Autodesk Inventor part; units mm, degrees
ref_plane "YZ Plane" through (0, 0, 0) normal (1, 0, 0) x (0, 1, 0)
ref_plane "XZ Plane" through (0, 0, 0) normal (0, 1, 0) x (-1, 0, 0)
ref_plane "XY Plane" through (0, 0, 0) normal (0, 0, 1) x (1, 0, 0)
sketch "Boceto1" plane through (0, 0, 0) normal (0, 0, 1) x (1, 0, 0)
  line L0 (0.15, 0) -> (0, 0)
  line L1 (0, 0) -> (0, 8.5)
  line L2 (0, 8.5) -> (0.15, 8.5)
  line L3 (0.15, 8.5) -> (0.15, 0)
  line L4 (0.15, 0) -> (5.9, 0)
  line L5 (5.9, 0) -> (5.9, 8.5)
  line L6 (5.9, 8.5) -> (5.75, 8.5)
  line L7 (5.75, 8.5) -> (5.6932, 0)
  line L8 (5.75, 8.5) -> (0.15, 8.5)
  circle A0 centre (0.5, 2.35) radius 0.15
  circle A1 centre (5.4, 2.35) radius 0.15
  circle A2 centre (0.5, 8.15) radius 0.15
  circle A3 centre (5.4, 8.15) radius 0.15
extrude "Extrusión1" add sketch "Boceto1" along normal blind 0.15
sketch "Boceto2" plane through (5.9, 0, 0) normal (1, 0, 0) x (0, 0, -1)
  line L0 (0, 0) -> (0, 8.5)
  line L1 (0, 8.5) -> (-0.8328, 8.5)
  line L2 (-0.8328, 8.5) -> (-0.8328, 0)
  line L3 (-0.8328, 0) -> (0, 0)
  circle A0 centre (-0.3164, 0.3) radius 0.15
  circle A1 centre (-0.3164, 1.2) radius 0.15
  line L4 (0, 8.5) -> (-0.15, 8.5)
  line L5 (-0.15, 8.5) -> (-0.15, 0)
extrude "Extrusión2" add sketch "Boceto2" against normal blind 0.15 contours L3 L2 L1 L5
sketch "Boceto3" plane through (0, 0, 0) normal (-1, 0, 0) x (0, 0, 1)
  line L0 (0, 0) -> (0, 8.5)
  line L1 (0, 8.5) -> (0.8328, 8.5)
  line L2 (0.8328, 8.5) -> (0.8328, 0)
  line L3 (0.8328, 0) -> (0, 0)
  circle A0 centre (0.3164, 0.3) radius 0.15
  circle A1 centre (0.3164, 1.2) radius 0.15
  line L4 (0, 8.5) -> (0.15, 8.5)
  line L5 (0.15, 8.5) -> (0.15, 0)
extrude "Extrusión3" add sketch "Boceto3" against normal blind 0.15 contours L5 L1 L2 L3
properties part number "learnbotAgarreOdroid"
Geometry: final body of the model. Coordinates: model frame, mm. Round coordinates to 2 decimals unless told otherwise and drop trailing zeros. Write each loop counter-clockwise with the first axis right and the second up, starting at its lowest first coordinate (ties: lowest second). Pieces come first, ordered by that corner, then holes. Notation, with made-up numbers: M 13.5,-34 L 49.5,-34 A27 ccw 49.5,-12 Z; hole C -6.5,38.25 d9. An arc over 180 degrees is marked long. Write item = value, one per line.
Item 1: Material intervals for line 1 along X through (y, z) = (2.5, 0.75); line 2 along Y through (x, z) = (5.4, 0.1); line 3 along Z through (x, y) = (0.7, 2.75), sorted ascending. Write a range as [from, to].
Findings:
line_1 = [0, 0.15], [5.75, 5.9]
line_2 = [0, 2.2], [2.5, 8], [8.3, 8.5]
line_3 = [0, 0.15]
Item 2: Section query B-B on x = 0.5. Return loops of the section in (y, z), then the cut area to 4 significant figures.
Findings:
outline = M 0,0 L 2.2,0 L 2.2,0.15 L 0,0.15 Z; M 2.5,0 L 8,0 L 8,0.15 L 2.5,0.15 Z; M 8.3,0 L 8.5,0 L 8.5,0.15 L 8.3,0.15 Z
area = 1.185 mm^2
Item 3: Section query C-C on y = 7. Return loops of the section in (x, z).
Findings:
outline = M 0,0 L 5.9,0 L 5.9,0.83 L 5.75,0.83 L 5.75,0.15 L 0.15,0.15 L 0.15,0.83 L 0,0.83 Z
Item 4: Section query A-A on y = 0.3. State how many separate pieces and enclosed holes the cut face has, then the cut area to 4 significant figures.
Findings:
separate_pieces = 3
enclosed_holes = 0
area = 1.000 mm^2
